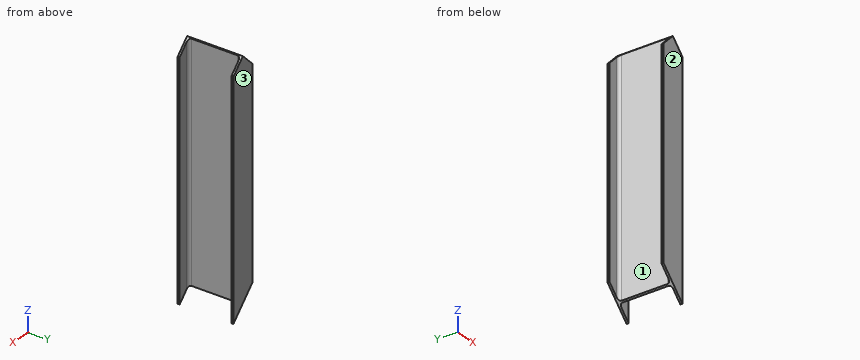
Autodesk Inventor part; units mm, degrees
ref_plane "Start Plane" through (0, 0, -85) normal (0, 0, 1) x (1, 0, 0)
ref_plane "End Plane" through (0, 0, 1500) normal (0, 0, 1) x (1, 0, 0)
ref_plane "Work Plane4" through (85, 0, 1585) normal (-0.7071, 0, 0.7071) x (0.7071, 0, 0.7071)
ref_plane "Start Plane" through (0, 0, -85) normal (0, 0, 1) x (1, 0, 0)
ref_plane "End Plane" through (0, 0, 1500) normal (0, 0, 1) x (1, 0, 0)
sketch "Sketch" plane through (0, 0, 0) normal (0, 0, 1) x (1, 0, 0)
  line L0 (-85, 167.3) -> (-22, 167.3)
  line L1 (-85, 180) -> (-85, 167.3)
  line L2 (85, 180) -> (-85, 180)
  line L3 (85, 167.3) -> (85, 180)
  line L4 (22, 167.3) -> (85, 167.3)
  line L5 (4, -149.3) -> (4, 149.3)
  line L6 (85, -167.3) -> (22, -167.3)
  line L7 (85, -180) -> (85, -167.3)
  line L8 (-85, -167.3) -> (-85, -180)
  line L9 (-22, -167.3) -> (-85, -167.3)
  line L10 (-4, 149.3) -> (-4, -149.3)
  line L11 (0, -252) -> (0, 252) construction
  line L12 (-4, -167.3) -> (4, -167.3) construction
  arc A0 (-22, -167.3) -> (-4, -149.3) centre (-22, -149.3) ccw
  arc A1 (-4, 149.3) -> (-22, 167.3) centre (-22, 149.3) ccw
  arc A2 (22, 167.3) -> (4, 149.3) centre (22, 149.3) ccw
  arc A3 (4, -149.3) -> (22, -167.3) centre (22, -149.3) ccw
  line L13 (-119, 0) -> (119, 0) construction
  line L14 (-85, -180) -> (85, -180)
  point P0 (-4, 167.3)
  point P1 (4, 167.3)
  point P2 (0, 0)
  point P3 (0, -167.3)
  point P4 (0, 0)
  dimension "d1" = 360
  dimension "d3" = 12.7
  dimension "d5" = 8
  dimension "d7" = 170
  dimension "d13" = 18
  dimension "d14" = 180
  dimension "d15" = 85
extrude "Body" add sketch "Sketch" along normal up to surface (1585 mm away) from surface at -85
sketch "Sketch3" plane through (0, 0, 0) normal (0, 0, 1) x (1, 0, 0)
  line L0 (0, 0) -> (10, 0)
ref_plane "Work Plane3" through (0, 0, 0) normal (0, -1, 0) x (1, 0, 0)
ref_plane "Work Plane4" through (85, 0, 1585) normal (-0.7071, 0, 0.7071) x (0.7071, 0, 0.7071)
split "Split1" plane through (85, 0, 1585) removes the side toward (-0.7071, 0, 0.7071)
ref_plane "Work Plane5" through (85, 0, -85) normal (-0.7071, 0, -0.7071) x (-0.7071, 0, 0.7071)
split "Split2" plane through (85, 0, -85) removes the side toward (-0.7071, 0, -0.7071)
ref_plane "Work Plane6" through (-85, 0, 1585) normal (0.7071, 0, 0.7071) x (0.7071, 0, -0.7071)
split "Split3" plane through (-85, 0, 1585) removes the side toward (0.7071, 0, 0.7071)
sketch "Sketch4" plane through (0, 0, 0) normal (0, -1, 0) x (1, 0, 0)
  line L0 (-2, -85) -> (12, -85)
  line L1 (-2, 1500) -> (12, 1500)
  dimension "d19" = 1585
equation "\"d1\" = ParH"
equation "\"d3\" = t2"
equation "\"d7\" = b"
equation "\"d13\" = R1"
equation "\"d14\" = 0.5 * d1"
equation "\"d15\" = 0.5 * d7"
equation "\"d8\" = G_L"
equation "\"b\" = 170"
equation "\"ParH\" = 360"
equation "\"R1\" = 18"
equation "\"G_L\" = d19"
equation "\"t1\" = 8"
equation "\"t2\" = 12.7"
equation "\"G_OFFSET_START\" = 85"
equation "\"G_OFFSET_END\" = 0"
equation "\"d16\" = -G_OFFSET_START"
properties part number "DIN 1025 - IPE 360-1585" material "Steel, Mild"
Part model, mm, in its own coordinate system. Face numbers are marked on the shaded views. Coordinates: 2 decimals unless noted, no trailing zeros. Loops run counter-clockwise (first coordinate to the right, second up) from the corner with the lowest first, then second, coordinate; pieces in that order, holes last. Notation, with made-up numbers: (26, -25.75) -> (51, -25.75) arc R33 ccw to (51, 6.25) -> close; hole circle Ø1 at (-11, 65). An arc over 180 degrees is marked (long way). Use a Markdown table: item, result. Add a question column.
Item 1: Probe probe 1 along Y at (x, z) = (55.5, 246.5); probe 2 along X at (y, z) = (-17, 1406.5); probe 3 along Y at (x, z) = (-7, 1281.5). List the from-to ranges inside material, lowest first.
Item 2: Band-saw the part on B-B on z = 138. Write the cut outline in (x, y).
Item 3: Pull direction Y, two halves, no side cores. Call the marked faces 1, 2 and 3: +Y half, -Y half, draft (parallel to the pull), parting line (faces both ways), or undercut.
Item 4: Band-saw the part on A-A on x = -68. Write the cut outline in (y, z), plus the area to 3 significant figures.
Item 5: Band-saw the part on C-C on x = 39. Write the cut outline in (y, z), plus the area to 3 significant figures.
Item 6: Flat gauge pins, fed straight in: P1, Ø5, axis at y = 18, z = 249.5, coming from the -X side; P2, Ø1, axis at x = 1, y = 7, coming from the -Z side; P3, Ø12, axis at y = 105.5, z = 823, coming from the +X side. Where does each tip first touch, or does it go through?
Item 7: Band-saw the part on D-D on y = -134. Write the cut outline in (x, z).
Geometry says:
| question | item | result |
|---|---|---|
| 1 | probe 1 | -180 to -167.3, 167.3 to 180 |
| 1 | probe 2 | -4 to 4 |
| 1 | probe 3 | -180 to -159.25, 159.25 to 180 |
| 2 | outline | (-85, -180) -> (85, -180) -> (85, -167.3) -> (22, -167.3) arc R18 cw to (4, -149.3) -> (4, 149.3) arc R18 cw to (22, 167.3) -> (85, 167.3) -> (85, 180) -> (-85, 180) -> (-85, 167.3) -> (-22, 167.3) arc R18 cw to (-4, 149.3) -> (-4, -149.3) arc R18 cw to (-22, -167.3) -> (-85, -167.3) -> close |
| 3 | face 1 | undercut |
| 3 | face 2 | -Y half |
| 3 | face 3 | +Y half |
| 4 | outline | (-180, 68) -> (-167.3, 68) -> (-167.3, 1432) -> (-180, 1432) -> close; (167.3, 68) -> (180, 68) -> (180, 1432) -> (167.3, 1432) -> close |
| 4 | area | 34,600 mm² |
| 5 | outline | (-180, -39) -> (-167.3, -39) -> (-167.3, 1461) -> (-180, 1461) -> close; (167.3, -39) -> (180, -39) -> (180, 1461) -> (167.3, 1461) -> close |
| 5 | area | 38,100 mm² |
| 6 | P1 | x = -4 |
| 6 | P2 | z = -1.5 |
| 6 | P3 | x = 4 |
| 7 | outline | (-4, 4) -> (4, -4) -> (4, 1496) -> (0, 1500) -> (-4, 1496) -> close |
